Answer from the drawing. Dimensions are ordinates in mm from the lowest x, y and z of the part. A direction names the side the tool comes from. Coordinates: 2 decimals unless noted, no trailing zeros. Write each loop counter-clockwise with the first axis right and the second up, starting at its lowest first coordinate (ties: lowest second). Pieces come first, ordered by that corner, then holes. Notation, with made-up numbers: M -6,79.25 L 16,79.25 A15 ccw 16,104.25 Z; hole C -19,67 d1. An arc over 180 degrees is marked long. Put each result on its own line as item: value. Start each with the question number.
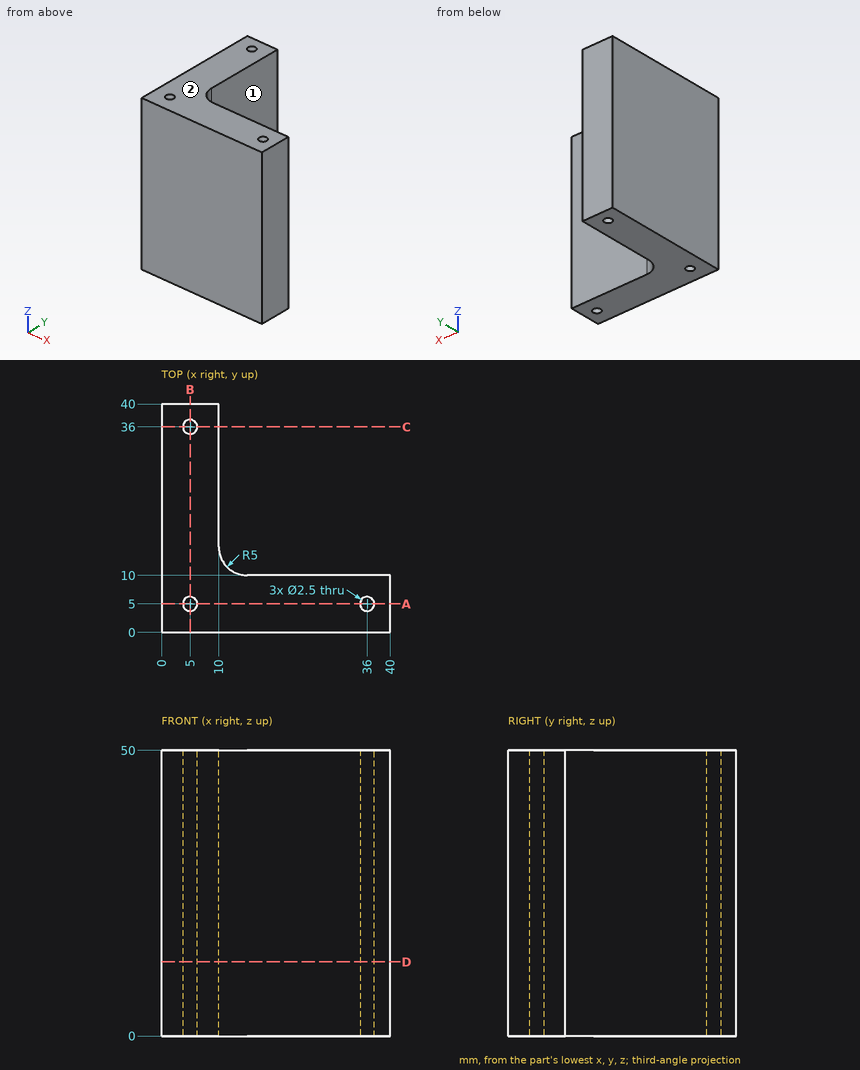
1) Given pin 1 Ø10 at (x, z) = (25, 37.5) entering from +Y; pin 2 Ø20 at (y, z) = (30.5, 20.5) entering from +X; pin 3 Ø2 at (x, y) = (5, 36) entering from -Z, each flat-ended and moving along its own axis, determine where each tip first touches the part or whether it passes through.
2) A cutting plane is placed at A-A on y = 5. Write down the section's boundary in (x, z).
3) For the marked faces 1 and 2, determine the directions among +Z, -Z, +X, -X, +Y, -Y from which every point of the face is accessible in a straight line to the end or side of a thin tool.
4) A cutting plane is placed at D-D on z = 13. Write down the section's boundary in (x, y).
5) Straight lines are drawn through the part: probe 1 along Y at (x, z) = (5, 11); probe 2 along Y at (x, z) = (6, 7). For each, find the intervals that lie inside material, in ascending order.
6) A cutting plane is placed at C-C on y = 36. Write down the section's boundary in (x, z).
Answers follow:
1. pin 1: stops at y = 10
1. pin 2: stops at x = 10
1. pin 3: passes through
2. outline: M 0,0 L 3.75,0 L 3.75,50 L 0,50 Z; M 6.25,0 L 34.75,0 L 34.75,50 L 6.25,50 Z; M 37.25,0 L 40,0 L 40,50 L 37.25,50 Z
3. face 1: +Z, -Z, +X, +Y
3. face 2: +Z, +X, -X, +Y, -Y
4. outline: M 0,0 L 40,0 L 40,10 L 15,10 A5 cw 10,15 L 10,40 L 0,40 Z; hole C 5,5 d2.5; hole C 5,36 d2.5; hole C 36,5 d2.5
5. probe 1: y = 0 to 3.75, 6.25 to 34.75, 37.25 to 40
5. probe 2: y = 0 to 4.25, 5.75 to 35.25, 36.75 to 40
6. outline: M 0,0 L 3.75,0 L 3.75,50 L 0,50 Z; M 6.25,0 L 10,0 L 10,50 L 6.25,50 Z
